Input: part model. Units: mm. Frame: model coordinates. Coordinates: 2 decimals unless noted, no trailing zeros. Loops run counter-clockwise (first coordinate to the right, second up) from the corner with the lowest first, then second, coordinate; pieces in that order, holes last. Notation, with made-up numbers: (-34.75, 74.25) - (4.25, 74.25) arc R11 cw to (4.25, 83.25) - close; hole circle Ø8 at (63.25, -37.5). An arc over 180 degrees is marked (long way). Use a Markdown table: item, result. Add a question column.
1. Draft query along Y for faces 1 (the face through (-16.276, -46.504, 4.93)), 2 (the face through (-15, 78.7, 4.9)), 3 (the face through (-24, 16, 0)). Return one class per face: released by +Y, released by -Y, zero draft, split by the parting line, or undercut.
2. Contact query for flat-ended pins moving along their axis: P1, Ø4, axis at x = -38, y = -64, coming from the -Z side; P2, Ø2, axis at x = -41, z = 3, coming from the -Y side; P3, Ø1, axis at x = -31.5, z = 4, coming from the +Y side; P4, Ø6, axis at x = -3.5, z = 7.5, coming from the +Y side. Output: stop coordinate, or through.
3. Section query B-B on x = -35. Return the cut outline in (y, z).
4. Section query C-C on y = 51.5. Return the cut outline in (x, z).
5. Ray query, L1, parallel to Y at x = 13.5, z = 6; L2, parallel to Y at x = -38.5, z = 3.25; L3, parallel to X at y = -48, z = 3.5. Return the intervals inside material, ascending. Write a range as [from, to].
6. Section query A-A on z = 7. Return the cut outline in (x, y), then the cut area to 3 significant figures.
```python
from build123d import *

# Parameters (mm, degrees)
F0_W     = 72.900745
F0_H     = 48.2
F1_DEPTH = 10


with BuildPart() as f1:
    # F0 (on Top) → F1 (new body)
    with BuildSketch(Plane.XY):
        with BuildLine():
            ThreePointArc((20.685012, 42.255733), (-15.765361, 78.706105), (-52.215733, 42.255733))
            Line((-52.215733, 42.255733), (20.685012, 42.255733))
        make_face()
        with Locations((-15.76536, 18.155733)):
            Rectangle(F0_W, F0_H)
        Polygon((20.685012, -5.944267), (-52.215733, -5.944267), (-52.215733, -85.944267), align=None)
    extrude(amount=F1_DEPTH)


solid = f1.part
```
Resolved:
| question | item | result |
|---|---|---|
| 1 | face 1 | released by -Y |
| 1 | face 2 | released by +Y |
| 1 | face 3 | zero draft |
| 2 | P1 | z = 0 |
| 2 | P2 | y = -74.73 |
| 2 | P3 | y = 75.37 |
| 2 | P4 | y = 77.51 |
| 3 | outline | (-67.05, 0) - (73.22, 0) - (73.22, 10) - (-67.05, 10) - close |
| 4 | outline | (-51.02, 0) - (19.49, 0) - (19.49, 10) - (-51.02, 10) - close |
| 5 | L1 | [-13.83, 63.99] |
| 5 | L2 | [-70.89, 70.75] |
| 5 | L3 | [-52.22, -17.64] |
| 6 | outline | (-52.22, -85.94) - (20.69, -5.94) - (20.69, 42.26) arc R36.45 ccw to (-52.22, 42.26) - close |
| 6 | area | 8,520 mm² |
